Source: three-view drawing plus pictorial views. Frame: mm from the lowest corner of the part. Give positions to 0.01 mm unless a question says otherwise; leave off trailing zeros. Write each loop counter-clockwise with the first axis right and the second up, starting at its lowest first coordinate (ties: lowest second). Pieces come first, ordered by that corner, then holes. Notation, with made-up numbers: (61, 42) -> (97, 42) arc R15 cw to (97, 54) -> close; hole circle Ø7 at (-38, 43.5). An arc over 180 degrees is marked (long way). Answer in a Markdown table with one row per item. Add a question column.
Item 1: Section query B-B on y = 7.5. Output: boundary loops of the cut face in (x, z), plus the area to 3 significant figures.
Item 2: Section query D-D on x = 2.75. Output: boundary loops of the cut face in (y, z), plus the area to 3 significant figures.
Item 3: Draft query along Y for the marked faces 1, 2 and 3. Return one class per face: +Y half, -Y half, draft (parallel to the pull), parting line (faces both ways), or undercut.
Item 4: First-contact query: P1, Ø8.5, axis at x = 9, y = 7.5, coming from the -Z side; P2, Ø4, axis at x = 9.5, y = 3.5, coming from the +Z side. Flat tips, straight axial feed; report the tip coordinate or a pass-through.
Item 5: Section query A-A on z = 0.2. Output: boundary loops of the cut face in (x, y).
Item 6: Material intervals for probe 1 along Y at (x, z) = (9, 1.25); probe 2 along Y at (x, z) = (11.5, 1.8); probe 3 along X at (y, z) = (7.25, 0.6), sorted ascending. Write a range as from..to.
Item 7: Section query C-C on x = 9. Output: boundary loops of the cut face in (y, z).
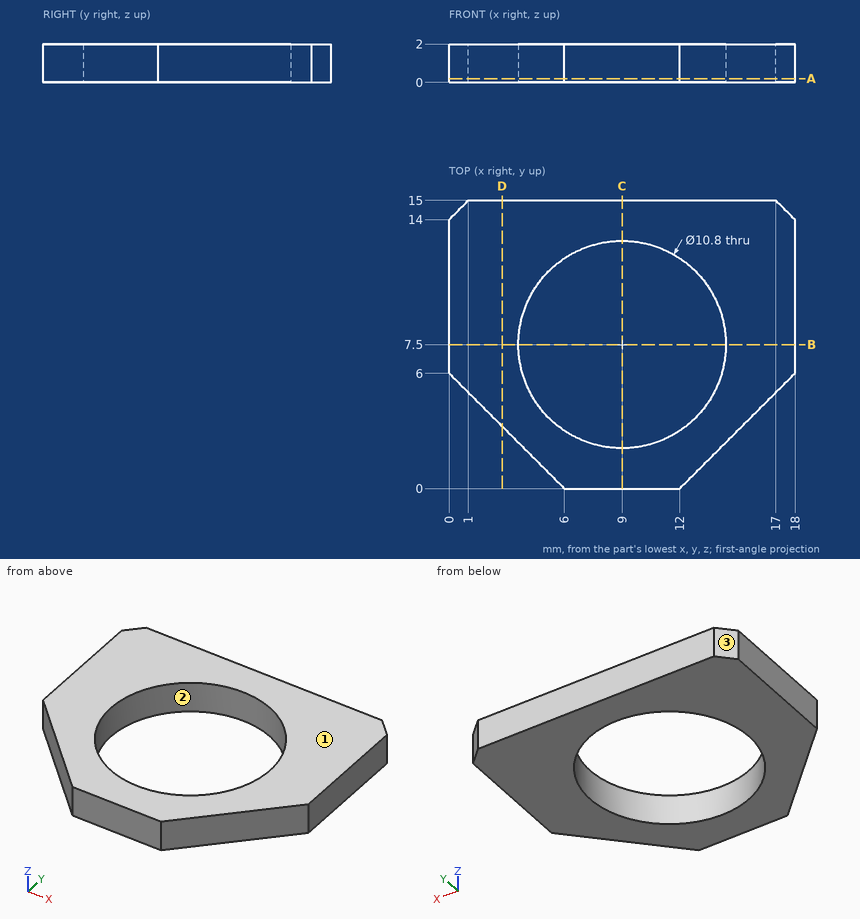
Findings below:
| question | item | result |
|---|---|---|
| 1 | outline | (0, 0) -> (3.6, 0) -> (3.6, 2) -> (0, 2) -> close; (14.4, 0) -> (18, 0) -> (18, 2) -> (14.4, 2) -> close |
| 1 | area | 14.4 mm^2 |
| 2 | outline | (3.25, 0) -> (15, 0) -> (15, 2) -> (3.25, 2) -> close |
| 2 | area | 23.5 mm^2 |
| 3 | face 1 | draft |
| 3 | face 2 | undercut |
| 3 | face 3 | +Y half |
| 4 | P1 | passes through |
| 4 | P2 | stops at z = 2 |
| 5 | outline | (0, 6) -> (6, 0) -> (12, 0) -> (18, 6) -> (18, 14) -> (17, 15) -> (1, 15) -> (0, 14) -> close; hole circle Ø10.8 at (9, 7.5) |
| 6 | probe 1 | y = 0..2.1, 12.9..15 |
| 6 | probe 2 | y = 0..2.71, 12.29..15 |
| 6 | probe 3 | x = 0..3.61, 14.39..18 |
| 7 | outline | (0, 0) -> (2.1, 0) -> (2.1, 2) -> (0, 2) -> close; (12.9, 0) -> (15, 0) -> (15, 2) -> (12.9, 2) -> close |
